Check sheet for the drawn part. Datum: minimum x, y, z corner. Units: mm. Give positions to 0.01 mm unless a question says otherwise; leave off trailing zeros. Order: outer loops, then holes, each group sorted by start corner. A loop starts at its lowest first (then second) coordinate and runs counter-clockwise, first axis right, second up. Notation, with made-up numbers: (68.5, -3) -> (121.5, -3) arc R18 ccw to (121.5, 28) -> close; hole circle Ø9 at (88.25, -1). An arc over 180 degrees is marked (long way). Return JSON: item names as keys, results as strings. Group by question number.
(1) Thickness scan on line 1 along Y through (x, z) = (29, 4.5); line 2 along X through (y, z) = (36.5, 6.25); line 3 along Y through (x, z) = (51, 2.25). Record the ranges inside material, lowest first.
(2) Cross-section at A-A on y = 29. Enter the section's corners in (x, z), then the cut area to 3 significant figures.
(3) Release check for a two-part mould opening along Y. For the marked faces 1, 2 and 3 record: pulls with the +Y half, pulls with the -Y half, needs draft (parallel to the pull), parting line crosses it, or undercut.
(4) Depth check by flat-ended pin: pin 1 Ø8 at (x, y) = (7.5, 23) entering from -Z; pin 2 Ø2 at (y, z) = (27, 5.5) entering from -X. Enter the tip coordinate at first touch or a pass-through.
(5) Cross-section at C-C on z = 5.25. Enter the section's corners in (x, y).
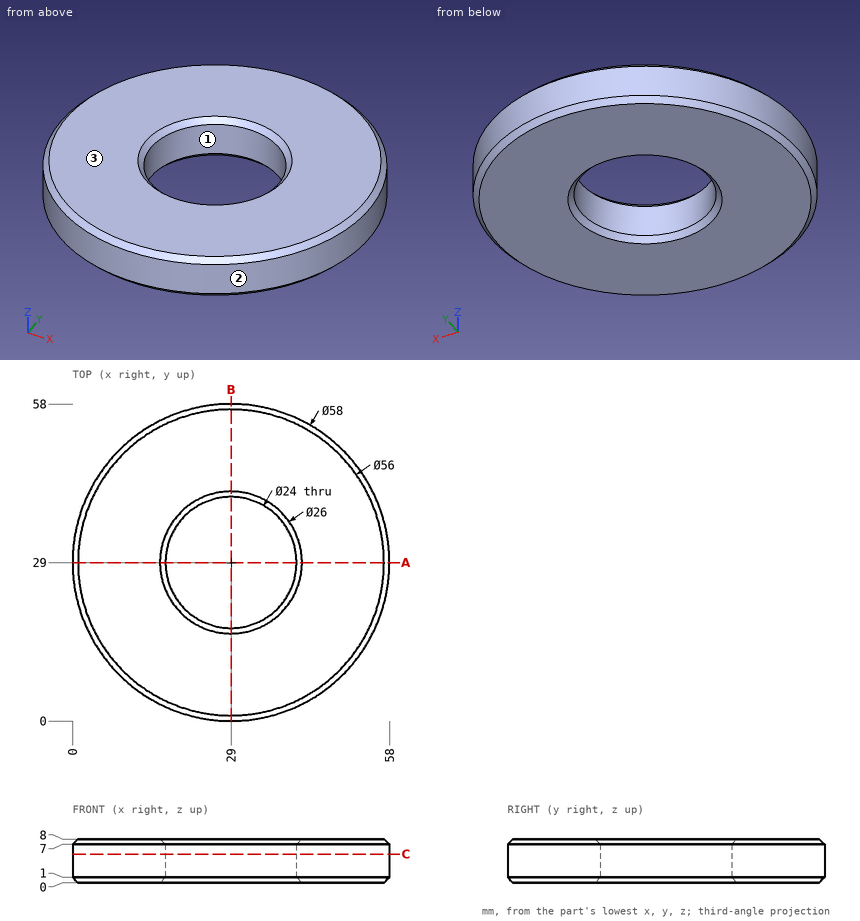
Verdict:
{
 "1": {"line 1": "0 to 17, 41 to 58", "line 2": "0.99 to 19.63, 38.37 to 57.01", "line 3": "10.11 to 47.89"},
 "2": {"outline": "(0, 1) -> (1, 0) -> (16, 0) -> (17, 1) -> (17, 7) -> (16, 8) -> (1, 8) -> (0, 7) -> close; (41, 1) -> (42, 0) -> (57, 0) -> (58, 1) -> (58, 7) -> (57, 8) -> (42, 8) -> (41, 7) -> close", "area": "268 mm²"},
 "3": {"face 1": "undercut", "face 2": "parting line crosses it", "face 3": "needs draft"},
 "4": {"pin 1": "z = 0", "pin 2": "x = 0.02"},
 "5": {"outline": "circle Ø58 at (29, 29); hole circle Ø24 at (29, 29)"}
}
